```python
from build123d import *

# Parameters (mm, degrees)
CUT_EXTRUDE1_DEPTH      = 113.342968182
CUT_EXTRUDE1_DEPTH_BACK = 113.342968182
SKETCH2_R               = 6.35
SKETCH3_R               = 3.175
CUT_EXTRUDE2_DEPTH      = 113.342968182
CIRPATTERN1_COUNT       = 8
SKETCH4_W               = 2.032
SKETCH4_H               = 2.54


with BuildPart() as part:
    # Sketch1 → Revolve1 (revolve)
    with BuildSketch(Plane.XY, mode=Mode.PRIVATE) as revolve1_sk:
        with BuildLine():
            Line((0, 76.2), (-10.16, 76.2))
            Line((-10.16, 76.2), (-10.16, 21.082))
            ThreePointArc((-10.16, 21.082), (-11.647897552, 17.489897552), (-15.24, 16.002))
            Line((-15.24, 16.002), (-31.75, 16.002))
            Line((-31.75, 16.002), (-31.75, 9.652))
            Line((-31.75, 9.652), (-6.35, 9.652))
            Line((-6.35, 9.652), (-6.35, 19.812))
            ThreePointArc((-6.35, 19.812), (-5.606051224, 21.608051224), (-3.81, 22.352))
            Line((-3.81, 22.352), (0, 22.352))
            Line((0, 22.352), (0, 76.2))
        make_face()
    revolve(revolve1_sk.sketch.rotate(Axis((0, 0, 0), (-1, 0, 0)), 90), axis=Axis((0, 0, 0), (-1, 0, 0)))

    # Sketch2 → Cut-Extrude1 (cut, two sides: drawn at the far end of the back side and taken through both)
    with BuildSketch(Plane(origin=(0, 0, 0), x_dir=(0, 0, -1), z_dir=(1, 0, 0)).offset(-CUT_EXTRUDE1_DEPTH_BACK)):
        with Locations((41.275, 0)):
            Circle(SKETCH2_R)
        with Locations((-41.275, 0)):
            Circle(SKETCH2_R)
    extrude(amount=CUT_EXTRUDE1_DEPTH + CUT_EXTRUDE1_DEPTH_BACK, mode=Mode.SUBTRACT)

    # Sketch3 → Cut-Extrude2 (cut, through all)
    with BuildSketch(Plane(origin=(0, 0, 0), x_dir=(0, 0, -1), z_dir=(1, 0, 0))):
        with Locations((66.802, 0)):
            Circle(SKETCH3_R)
    cut_extrude2 = extrude(amount=-CUT_EXTRUDE2_DEPTH, mode=Mode.SUBTRACT)

    # CirPattern1: Cut-Extrude2 ×8 about axis
    cirpattern1_axis = Axis((0, 0, 0), (1, 0, 0))
    for i in range(1, CIRPATTERN1_COUNT):
        add(cut_extrude2.rotate(cirpattern1_axis, i * 360 / CIRPATTERN1_COUNT), mode=Mode.SUBTRACT)

    # Sketch4 → Cut-Revolve1 (revolve, cut)
    with BuildSketch(Plane.XY):
        with Locations((-1.016, 24.892)):
            Rectangle(SKETCH4_W, SKETCH4_H)
    revolve(axis=Axis((0, 0, 0), (-1, 0, 0)), mode=Mode.SUBTRACT)


solid = part.part
```
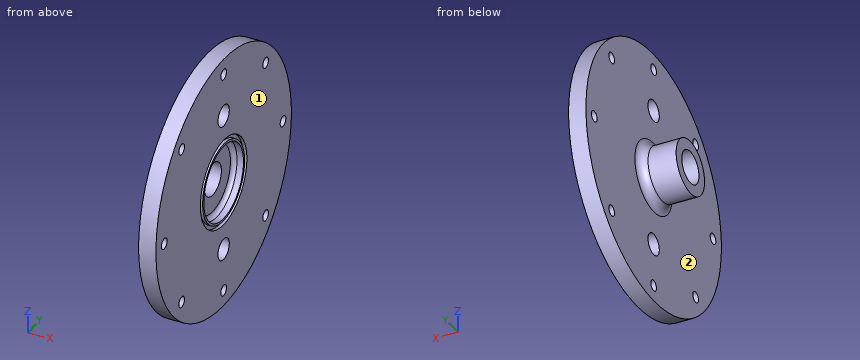
Part model, mm, in its own coordinate system. Face numbers are marked on the shaded views. A direction names the side the tool comes from. Give positions to 0.01 mm unless a question says otherwise; leave off trailing zeros. Write each loop counter-clockwise with the first axis right and the second up, starting at its lowest first coordinate (ties: lowest second). Pieces come first, ordered by that corner, then holes. Notation, with made-up numbers: (83.5, -39) -> (87.5, -39) arc R23 ccw to (87.5, -18) -> close; hole circle Ø3 at (80, -5.5). An arc over 180 degrees is marked (long way). Put each result on its own line as item: value. Start each with the question number.
Item 1: Which spindle directions (+Z, -Z, +X, -X, +Y, -Y) get a long thin tool onto all of the face, cutting with end or side? Do the marked faces 1 and 2. Say none if no direction does.
Item 2: Wall check: L1, parallel to X at y = 44.5, z = -11.5; L2, parallel to Y at x = -3.5, z = -15; L3, parallel to Z at x = -15.5, y = 8.5. Give the ranges that are in metal, low to high. Write a range as [from, to].
Item 3: Cut at C-C (x = -22). List the corners of the cut face in (y, z).
Item 4: Cut at A-A (y = 0). State how many separate pieces and enclosed holes the cut face has, then the cut area to 3 significant figures.
Item 5: Pin check, flat tips, straight feed: pin 1 Ø16.5 at (y, z) = (0, 41.275) entering from -X; pin 2 Ø1.5 at (x, y) = (-8, -8.5) entering from -Z; pin 3 Ø12 at (y, z) = (-6, 1.5) entering from +X; pin 4 Ø5.5 at (y, z) = (47.24, 47.24) entering from +X. Stop position of each tip, or through.
Item 6: Cut at D-D (y = 56). List the corners of the cut face in (x, z).
Answer list:
1. face 1: +Z, -Z, +X, +Y, -Y
1. face 2: -X
2. L1: x = [-10.16, 0]
2. L2: y = [-74.71, -16.57], [16.57, 74.71]
2. L3: z = [-13.56, -4.57], [4.57, 13.56]
3. outline: circle Ø32 at (0, 0); hole circle Ø19.3 at (0, 0)
4. separate pieces: 6
4. enclosed holes: 0
4. area: 1,080 mm2
5. pin 1: stops at x = -10.16
5. pin 2: stops at z = -75.8
5. pin 3: stops at x = -6.35
5. pin 4: passes through
6. outline: (-10.16, -51.68) -> (0, -51.68) -> (0, 51.68) -> (-10.16, 51.68) -> close
